Check sheet for the modelled part. Datum: model origin and axes. Units: mm. Give positions to 0.01 mm unless a question says otherwise; leave off trailing zeros. Loops run counter-clockwise (first coordinate to the right, second up) from the corner with the lowest first, then second, coordinate; pieces in that order, holes last.
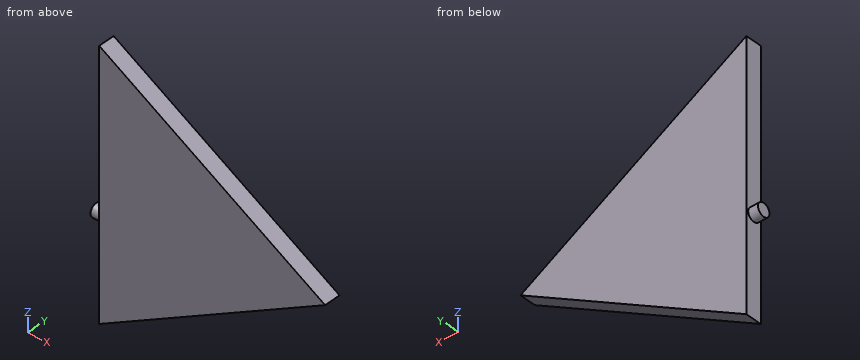
```python
from build123d import *

# Parameters (mm, degrees)
BOSS_EXTRUDE1_DEPTH = 5
SKETCH2_R           = 2
BOSS_EXTRUDE2_DEPTH = 3


with BuildPart() as part:
    # Sketch1 → Boss-Extrude1 (new body)
    with BuildSketch(Plane(origin=(0, 0, 0), x_dir=(1, 0, 0), z_dir=(0, 1, 0))):
        Polygon((-69.282032303, 40), (0, 0), (-69.282032303, -40), align=None)
    extrude(amount=BOSS_EXTRUDE1_DEPTH)

    # Sketch2 → Boss-Extrude2 (add)
    with BuildSketch(Plane.ZY.offset(69.282032303)):
        with Locations((-10, 2.360160214)):
            Circle(SKETCH2_R)
    extrude(amount=BOSS_EXTRUDE2_DEPTH)


solid = part.part
```
(1) Material ranges on line 1 (Z direction, x = -10, y = 3.85); line 2 (X direction, y = 1.85, z = -36); line 3 (Z direction, x = -11.5, y = 1.35), recorded low to high.
(2) Section check C-C on x = -39.5. Record the boundary of the cut face in (y, z), plus the area to 3 significant figures.
(3) Gauge pin test, flat ends, axial feed: pin 1 Ø2 at (x, y) = (-8, 2.5) entering from -Z; pin 2 Ø1.5 at (y, z) = (2, 11.5) entering from -X; pin 3 Ø1 at (x, y) = (-15.5, 2) entering from +Z. Record the tip position at first contact, or that the pin passes through.
(4) Section check B-B on z = -11. Record the boundary of the cut face in (x, y).
(5) Section check A-A on y = 3.6. Record the boundary of the cut face in (x, z).
(6) Section check D-D on z = -30. Record the boundary of the cut face in (x, y).
Computed values:
1. line 1: z = -5.77 to 5.77
1. line 2: x = -69.28 to -62.35
1. line 3: z = -6.64 to 6.64
2. outline: (0, -22.81) - (5, -22.81) - (5, 22.81) - (0, 22.81) - close
2. area: 228 mm2
3. pin 1: stops at z = -5.2
3. pin 2: stops at x = -69.28
3. pin 3: stops at z = 9.24
4. outline: (-72.28, 0.63) - (-69.28, 0.63) - (-69.28, 0) - (-19.05, 0) - (-19.05, 5) - (-69.28, 5) - (-69.28, 4.09) - (-72.28, 4.09) - close
5. outline: (-72.28, -11.57) - (-69.28, -11.57) - (-69.28, -40) - (0, 0) - (-69.28, 40) - (-69.28, -8.43) - (-72.28, -8.43) - close
6. outline: (-69.28, 0) - (-51.96, 0) - (-51.96, 5) - (-69.28, 5) - close
